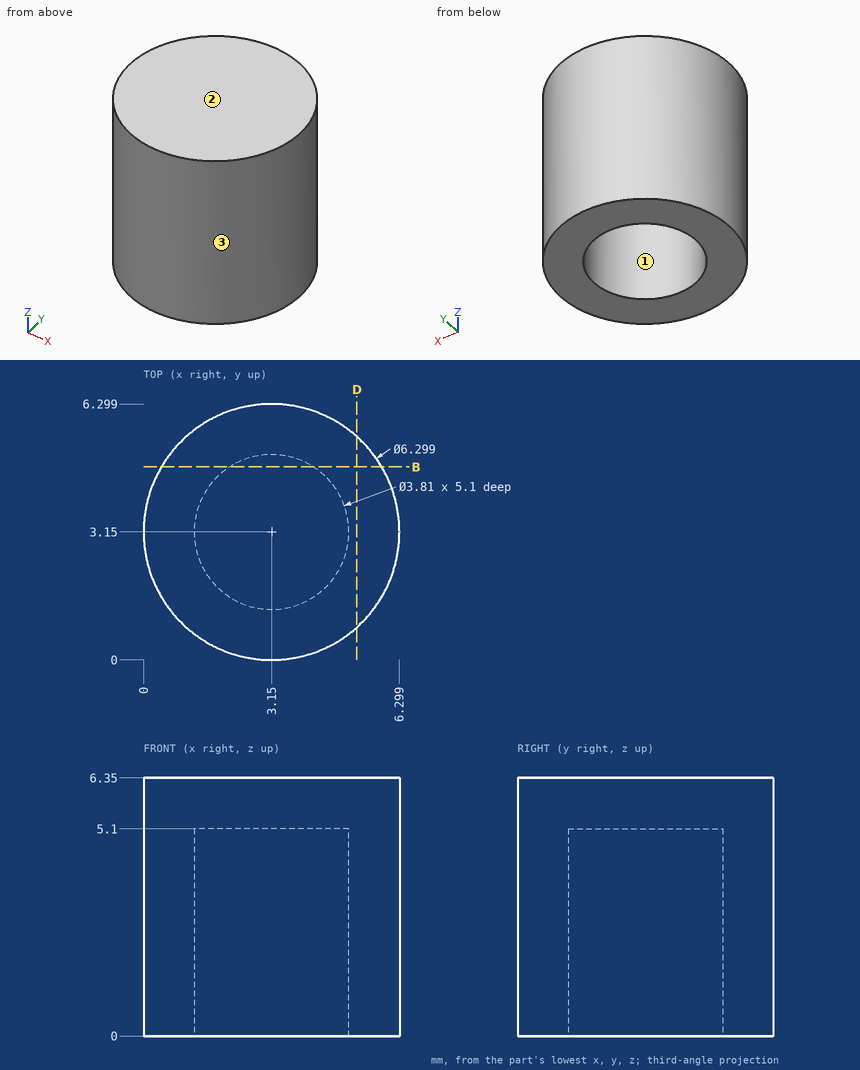
Input: dimensioned drawing with shaded views. Units: mm. Origin: part minimum x, y, z. Give positions to 0.01 mm unless a question says otherwise; leave off trailing zeros. Write each loop counter-clockwise with the first axis right and the second up, starting at its lowest first coordinate (ties: lowest second). Pieces come first, ordered by that corner, then holes. Notation, with made-up numbers: (-37.5, 84) -> (16.5, 84) arc R33 ccw to (16.5, 113) -> close; hole circle Ø4 at (-37.5, 1.5). An arc over 180 degrees is marked (long way). Answer as a JSON object with one key per item and string values.
1. Contact query for flat-ended pins moving along their axis: pin 1 (1.9 mm diameter, centred on x = 2.5, y = 4, fed in from -Z); pin 2 (2 mm diameter, centred on x = 2, z = 1, fed in from -Y); pin 3 (1 mm diameter, centred on x = 1, z = 3.5, fed in from +Y). Output: stop coordinate, or through.
Ans:
{"pin 1": "stops at z = 0", "pin 2": "stops at y = 0", "pin 3": "stops at y = 5.83"}
2. Cut plane D-D on x = 5.25. Output: boundary loops of the cut face in (y, z), and give its area (3 significant figures).
Ans:
{"outline": "(0.8, 0) -> (5.5, 0) -> (5.5, 6.35) -> (0.8, 6.35) -> close", "area": "29.8 mm^2"}
3. Ray query, probe 1 along Y at (x, z) = (3.25, 2.5); probe 2 along Z at (x, y) = (4, 2.25); probe 3 along Y at (x, z) = (2, 4.25). Return the intervals inside material, ascending. Write a range as from..to.
Ans:
{"probe 1": "y = 0..1.25, 5.05..6.3", "probe 2": "z = 5.1..6.35", "probe 3": "y = 0.22..1.63, 4.67..6.08"}
4. Mould query, pull axis X, two halves, no side actions, for the marked faces 1, 2 and 3. Classes: pulls with the +X half, pulls with the -X half, needs draft (parallel to the pull), parting line crosses it, or undercut.
Ans:
{"face 1": "undercut", "face 2": "needs draft", "face 3": "parting line crosses it"}
5. Cut plane B-B on y = 4.75. Output: boundary loops of the cut face in (x, z), and give its area (3 significant figures).
Ans:
{"outline": "(0.44, 0) -> (2.12, 0) -> (2.12, 5.1) -> (4.18, 5.1) -> (4.18, 0) -> (5.86, 0) -> (5.86, 6.35) -> (0.44, 6.35) -> close", "area": "23.9 mm^2"}
